Autodesk Inventor part; units mm, degrees
ref_plane "Work Plane1" through (1.525, 0, 0) normal (0, 0, 1) x (1, 0, 0)
ref_plane "YZ Plane" through (0, 0, 0) normal (1, 0, 0) x (0, 1, 0)
ref_plane "XZ Plane" through (0, 0, 0) normal (0, 1, 0) x (-1, 0, 0)
sketch "Skizze1" plane through (0, 0, 0) normal (0, 0, 1) x (1, 0, 0)
  line L0 (0, 6) -> (60, 6)
  line L1 (60, 6) -> (60, 0)
  line L2 (60, 0) -> (0, 0)
  line L3 (-12, 0) -> (72, 0)
  line L4 (0, -1.2) -> (0, 7.2)
  line L5 (0, 6) -> (0, 0)
  dimension "d2" = 12
  dimension "d59" = 60
revolve "Körper" add sketch "Skizze1" angle 360 about axis through (60, 0, 0) along (-1, 0, 0)
sketch "Skizze2" plane through (0, 0, 0) normal (-1, 0, 0) x (0, 0, 1)
  line L0 (0, 9.815) -> (8.5, 4.9075)
  line L1 (8.5, 4.9075) -> (8.5, -4.9075)
  line L2 (8.5, -4.9075) -> (0, -9.815)
  line L3 (0, -9.815) -> (-8.5, -4.9075)
  line L4 (-8.5, -4.9075) -> (-8.5, 4.9075)
  line L5 (-8.5, 4.9075) -> (0, 9.815)
  line L6 (-11.9, 0) -> (11.9, 0)
  line L7 (0, 13.7409) -> (0, -13.7409)
  point P0 (0, 0)
  point P1 (0, 0)
  dimension "d11" = 17
extrude "Kopf" add sketch "Skizze2" along normal blind 7.5
sketch "Skizze4" plane through (0, 0, 0) normal (0, 0, 1) x (1, 0, 0)
  line L0 (-6.5185, 10.2) -> (-7.5, 8.5)
  line L1 (-1.1, 0) -> (-0.234, 0)
  line L2 (-8.9532, 0) -> (1.2192, 0)
  line L3 (-7.5, 10.2) -> (-6.5185, 10.2)
  line L4 (-7.5, 8.5) -> (-7.5, 10.2)
  line L5 (0, 12.24) -> (0, -2.04)
  dimension "d65" = 17
  dimension "d67" = 30
  dimension "d68" = 20.4
  dimension "d69" = 7.5
revolve "Fase1" cut sketch "Skizze4" angle 360 about axis through (-1.1, 0, 0) along (1, 0, 0)
thread "Gewinde"
chamfer "Fase2" distance 1.0735 distance2 1.0736 1 edges at (60, -6, 0) measured on face at (60, -2.1318, 1.2492)
fillet "Fillet2" radius 0.1 1 edges at (0, -6, 0)
ref_plane "Work Plane1" through (1.525, 0, 0) normal (0, 0, 1) x (1, 0, 0)
equation "\"d2\" = GD"
equation "\"d59\" = NLG"
equation "\"d11\" = SW"
equation "\"d3\" = KOH"
equation "\"d71\" = RR"
equation "\"d15\" = GEL"
equation "\"d6\" = -0.5 * SPD + 0.5 * GD"
equation "\"d65\" = SW"
equation "\"d67\" = ANG1"
equation "\"d68\" = 1.2 * SW"
equation "\"d69\" = KOH"
equation "\"NLG\" = 60"
equation "\"GD\" = NND"
equation "\"BDM\" = NND"
equation "\"KOH\" = 7.5"
equation "\"GEL\" = 30"
equation "\"SW\" = 17"
equation "\"SW0\" = SW"
equation "\"SPD\" = NND - 1.2269 * PTC"
equation "\"SD2\" = NND"
equation "\"SD\" = 0"
equation "\"ANG1\" = 30deg"
equation "\"GAL\" = 0.61345 * PTC"
equation "\"GUL\" = 0.61345 * PTC"
equation "\"RR\" = 0.1"
equation "\"RR1\" = 0.1"
equation "\"GD1\" = THREADDIA - 1.2269 * PTC"
equation "\"THREADDIA\" = 12"
equation "\"TOA\" = 30deg"
equation "\"PTC\" = 1.75"
equation "\"NND\" = 12"
equation "\"E0\" = 1.155 * SW"
properties part number "ISO 4016 - M12 x 60" material "Steel, Mild"
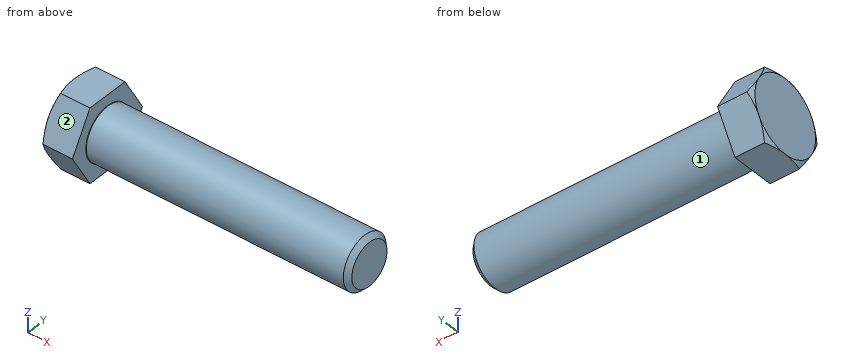
CAD build for the part. Positions are in the model's coordinates, mm. Face numbers are marked on the shaded views. A direction names the side the tool comes from. Round coordinates to 2 decimals unless told otherwise and drop trailing zeros. Write each loop counter-clockwise with the first axis right and the second up, starting at its lowest first coordinate (ties: lowest second). Pieces come first, ordered by that corner, then holes. Notation, with made-up numbers: (28.5, 50) -> (32.5, 50) arc R5 ccw to (32.5, 56) -> close; hole circle Ø10 at (-38.75, -31.75). An arc over 180 degrees is marked (long way). Answer in a Markdown table with one row per item. Add a question column.
Item 1: Drill centre lines: line 1 (X direction, y = -3.75, z = 6); line 2 (Z direction, x = 37, y = 0.25). Where is each one in solid material? Low to high. Write a range as from..to.
Item 2: Saw through at A-A, the plane x = 15. Write the cut outline in (y, z).
Item 3: Which spindle directions (+Z, -Z, +X, -X, +Y, -Y) get a long thin tool onto all of the face, cutting with end or side? Do the marked faces 1 and 2. Say none if no direction does.
Item 4: Drop flat-ended pins along their axis: pin 1 Ø4 at (x, z) = (20, 6) entering from +Y; pin 2 Ø5 at (x, z) = (52.5, 6.5) entering from -Y; pin 3 Ø10 at (x, z) = (15.5, 0) entering from -Y. Give the stop position or say it passes through.
Findings below:
| question | item | result |
|---|---|---|
| 1 | line 1 | x = -7.5..0 |
| 1 | line 2 | z = -5.99..5.99 |
| 2 | outline | circle Ø12 at (0, 0) |
| 3 | face 1 | +X |
| 3 | face 2 | +Z, +X, -X, -Y |
| 4 | pin 1 | stops at y = 4.47 |
| 4 | pin 2 | stops at y = -4.47 |
| 4 | pin 3 | stops at y = -6 |
